Model file for the job. Use its own axes, mm. A direction names the side the tool comes from. Give positions to 0.01 mm unless a question says otherwise; leave off trailing zeros. Loops run counter-clockwise (first coordinate to the right, second up) from the corner with the lowest first, then second, coordinate; pieces in that order, holes last. Notation, with made-up numbers: M -15,2 L 5,2 A30 ccw 5,35 Z; hole C 89,46.25 d8. An arc over 180 degrees is marked long. Answer in a Markdown table with one row per item.
```python
from build123d import *

# Parameters (mm, degrees)
EXTRUDE_THIN1_DEPTH            = 1125.4359
F_4_CLEARANCE_HOLE1_AT_2_COUNT = 2
F_4_CLEARANCE_HOLE1_AT_2_PITCH = 450


with BuildPart() as part:
    # Sketch1 → Extrude-Thin1 (new body)
    with BuildSketch(Plane.XY):
        Polygon((-38.1, 0), (0, 0), (0, -19.05), (-1.5748, -19.05), (-1.5748, -1.5748), (-38.1, -1.5748), align=None)
    extrude(amount=EXTRUDE_THIN1_DEPTH)

    # Sketch2 → #4 Clearance Hole1 (revolve, cut)
    with BuildSketch(Plane(origin=(-20.32, 0, 15.875), x_dir=(0, 0, 1), z_dir=(1, 0, 0))):
        Polygon((0, 0), (0, 1.5748), (2.1082, 1.5748), (1.4732, 0.9398), (1.4732, 0.635), (2.1082, 0), align=None)
    f_4_clearance_hole1 = revolve(axis=Axis((-20.32, 6.35, 15.875), (0, -1, 0)), mode=Mode.SUBTRACT)

    # #4 Clearance Hole1 at 2: #4 Clearance Hole1 ×2
    with Locations(*[(0, 0, i * F_4_CLEARANCE_HOLE1_AT_2_PITCH) for i in range(1, F_4_CLEARANCE_HOLE1_AT_2_COUNT)]):
        add(f_4_clearance_hole1, mode=Mode.SUBTRACT)


solid = part.part
```
(1) Saw through at B-B, the plane y = -10.25. Give the cut face in (x, z), and give its area (3 significant figures).
Established:
| item | result |
|---|---|
| outline | M -1.57,0 L 0,0 L 0,1125.44 L -1.57,1125.44 Z |
| area | 1,770 mm2 |
(2) Flat gauge pins, fed straight in: P1, Ø3, axis at y = -11, z = 644, coming from the -X side; P2, Ø1.5, axis at x = -28, y = -2.5, coming from the -Z side; P3, Ø3.5, axis at x = -20.32, z = 15.875, coming from the -Y side. Where does each tip first touch, or does it go through?
Established:
| item | result |
|---|---|
| P1 | stops at x = -1.57 |
| P2 | passes through |
| P3 | stops at y = -1.22 |
(3) Wall check: L1, parallel to Z at x = -20.32, y = -0.8; L2, parallel to X at y = -14, z = 712. Give the ranges that are in metal, low to high.
Established:
| item | result |
|---|---|
| L1 | z = 0 to 14.4, 17.35 to 464.4, 467.35 to 1125.44 |
| L2 | x = -1.57 to 0 |
(4) Saw through at A-A, the plane z = 761. Give the cut face in (x, y), and give its area (3 significant figures).
Established:
| item | result |
|---|---|
| outline | M -38.1,-1.57 L -1.57,-1.57 L -1.57,-19.05 L 0,-19.05 L 0,0 L -38.1,0 Z |
| area | 87.5 mm2 |
(5) Which spindle directions (+Z, -Z, +X, -X, +Y, -Y) get a long thin tool onto all of the face, cutting with end or side? Do faces 1 (the flat face through (-20, -1.575, 555)), 2 (the flat face through (0, -9, 555)). Say none if no direction does.
Established:
| item | result |
|---|---|
| face 1 | +Z, -Z, -X, -Y |
| face 2 | +Z, -Z, +X, +Y, -Y |
